Build history of the part. All positions in model axes, mm. Give positions to 0.01 mm unless a question says otherwise; leave off trailing zeros. Write each loop counter-clockwise with the first axis right and the second up, starting at its lowest first coordinate (ties: lowest second). Pieces come first, ordered by that corner, then holes. Notation, with made-up numbers: M 16,29 L 54,29 A26 ccw 54,43 Z; hole C 86.25,33 d10. An arc over 180 degrees is marked long. Return JSON: item names as keys, results as strings. Group by question number.
Q1. Flat gauge pins, fed straight in: pin 1 Ø1.5 at (x, y) = (22, 220) entering from -Z; pin 2 Ø4 at (x, z) = (25, 5) entering from +Y; pin 3 Ø8 at (x, z) = (10, 10.5) entering from +Y; pin 4 Ø10 at (x, z) = (45, 9.5) entering from -Y. Where does each tip first touch, or does it go through?
Q2. Band-saw the part on A-A, the plane x = 25. Give the cut face in (y, z) (3 decimals), then the cut area to 3 significant figures.
Q3. Band-saw the part on B-B, the plane z = 5.75. Give the cut face in (x, y), then the cut area to 3 significant figures.
Q4. Wall check: probe 1 along Y at (x, z) = (25, 11.75); probe 2 along X at (y, z) = (480, 14); probe 3 along Y at (x, z) = (28.5, 9). Give the ranges that are in metal, low to high.
Q5. Pull direction Y, two halves, no side cores. Call faces 1 (the cylindrical face through (25.55, -24.994, 9.86)), 2 (the flat face through (50, 243, 10)), 3 (the cylindrical face through (25.651, 484.957, 9.848)): +Y half, -Y half, draft (parallel to the pull), parting line (faces both ways), or undercut.
from build123d import *

# Parameters (mm, degrees)
BOSS_EXTRUDE1_DEPTH              = 20
F_10_0MM_DOWEL_HOLE1_D           = 10
F_10_0MM_DOWEL_HOLE1_DEPTH       = 20
F_10_0MM_DOWEL_HOLE1_CSINK_D     = 10.05
F_10_0MM_DOWEL_HOLE1_CSINK_ANGLE = 90


with BuildPart() as part:
    # Sketch1 → Boss-Extrude1 (new body)
    with BuildSketch(Plane.XY):
        with BuildLine():
            Line((0, 0), (0, 480))
            ThreePointArc((0, 480), (25, 505), (50, 480))
            Line((50, 480), (50, 0))
            ThreePointArc((50, 0), (25, -25), (0, 0))
        make_face()
    extrude(amount=BOSS_EXTRUDE1_DEPTH)

    # Ø10.0mm Dowel Hole1
    with Locations(Plane.XY.offset(20)):
        with Locations((25, 480), (25, 0)):
            CounterSinkHole(F_10_0MM_DOWEL_HOLE1_D / 2, F_10_0MM_DOWEL_HOLE1_CSINK_D / 2, depth=F_10_0MM_DOWEL_HOLE1_DEPTH, counter_sink_angle=F_10_0MM_DOWEL_HOLE1_CSINK_ANGLE)


solid = part.part
From the geometry:
{
 "1": {"pin 1": "stops at z = 0", "pin 2": "stops at y = 505", "pin 3": "stops at y = 502.45", "pin 4": "stops at y = -20"},
 "2": {"outline": "M -25,0 L -5,0 L -5,19.975 L -5.025,20 L -25,20 Z; M 5,0 L 475,0 L 475,19.975 L 474.975,20 L 5.025,20 L 5,19.975 Z; M 485,0 L 505,0 L 505,20 L 485.025,20 L 485,19.975 Z", "area": "10,200 mm^2"},
 "3": {"outline": "M 0,0 A25 ccw 50,0 L 50,480 A25 ccw 0,480 Z; hole C 25,0 d10; hole C 25,480 d10", "area": "25,800 mm^2"},
 "4": {"probe 1": "y = -25 to -5, 5 to 475, 485 to 505", "probe 2": "x = 0 to 20, 30 to 50", "probe 3": "y = -24.75 to -3.57, 3.57 to 476.43, 483.57 to 504.75"},
 "5": {"face 1": "-Y half", "face 2": "draft", "face 3": "undercut"}
}
